The listing builds one solid part. Answer for the finished solid, in the listing's coordinates (mm). Coordinates: 2 decimals unless noted, no trailing zeros. Order: outer loops, then holes, each group sorted by start corner. A loop starts at its lowest first (then second) coordinate and runs counter-clockwise, first axis right, second up. Notation, with made-up numbers: (-21, 89.5) -> (-4, 89.5) arc R11 cw to (-4, 96.5) -> close; hole circle Ø8 at (57.5, 43.5). An arc over 180 degrees is marked (long way). One line per question, with ' | ' between items.
from build123d import *

# Parameters (mm, degrees)
F0_W     = 50.8
F0_H     = 19.05
F1_DEPTH = 1123.95
F2_W     = 122.435573
F2_H     = 50.8
F2_W_2   = 108.831619
F2_W_3   = 93.867282
F2_W_4   = 145.562325
F2_W_5   = 343.160421
F2_W_6   = 239.549167
F3_DEPTH = 25.4
F4_R     = 4.7625
F5_DEPTH = 25.4


with BuildPart() as f1:
    # F0 (on Top) → F1 (new body)
    with BuildSketch(Plane.XY):
        Rectangle(F0_W, F0_H)
    extrude(amount=F1_DEPTH)

    # F2 (on Front) → F3 (cut)
    with BuildSketch(Plane.XZ):
        with Locations((22.446524, 25.4)):
            Rectangle(F2_W, F2_H)
        with Locations((-4.761385, 342.9)):
            Rectangle(F2_W_2, F2_H)
        with Locations((2.720783, 755.65)):
            Rectangle(F2_W_3, F2_H)
        with Locations((-1.360391, 444.5)):
            Rectangle(F2_W_4, F2_H)
        with Locations((-38.781822, 1098.55)):
            Rectangle(F2_W_5, F2_H)
        with Locations((-25.794175, 254)):
            Rectangle(F2_W_6, F2_H)
    extrude(amount=F3_DEPTH, mode=Mode.SUBTRACT)

    # F4 (on Front) → F5 (cut)
    with BuildSketch(Plane.XZ):
        with Locations((15.875, 254)):
            Circle(F4_R)
        with Locations((15.875, 482.6)):
            Circle(F4_R)
    extrude(amount=F5_DEPTH, mode=Mode.SUBTRACT)


solid = f1.part
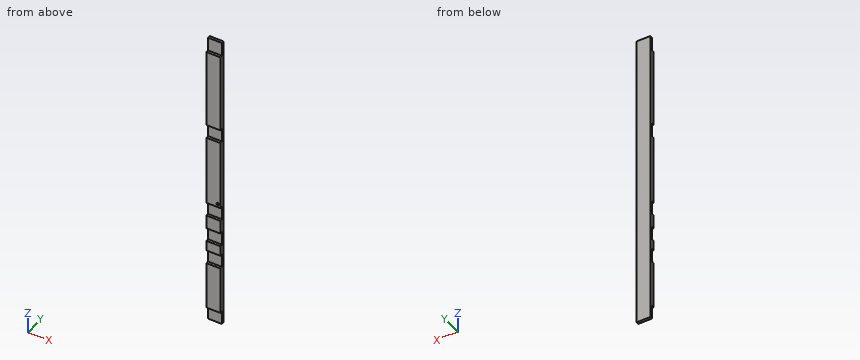
Item 1: Each of these flat-tipped pins is pushed along its axis until it touches: pin 1 Ø4 at (x, y) = (16.5, -4) entering from -Z; pin 2 Ø2 at (x, z) = (-18.5, 430) entering from -Y; pin 3 Ø3 at (x, y) = (12.5, -7) entering from +Z. Where does it stop, or does it pass through?
Computed values:
pin 1: stops at z = 50.8 | pin 2: stops at y = 0 | pin 3: stops at z = 1073.15
Item 2: Section A-A, the plane y = -5.25 is taken. Count the separate pieces of the cut face and the enclosed holes in it, plus the area to 3 significant figures.
Computed values:
separate pieces: 5 | enclosed holes: 1 | area: 41,500 mm^2
Item 3: Section C-C, the plane z = 752.5 is taken. Give the vertices of the cut face in (x, y) (3 decimals).
Computed values:
outline: (-25.4, 0) -> (25.4, 0) -> (25.4, 9.525) -> (-25.4, 9.525) -> close
Item 4: Section B-B, the plane x = -17 is taken. Give the vertices of the cut face in (y, z) (3 decimals), plus the area to 3 significant figures.
Computed values:
outline: (-9.525, 50.8) -> (0, 50.8) -> (0, 0) -> (9.525, 0) -> (9.525, 1123.95) -> (0, 1123.95) -> (0, 1073.15) -> (-9.525, 1073.15) -> (-9.525, 781.05) -> (0, 781.05) -> (0, 730.25) -> (-9.525, 730.25) -> (-9.525, 469.9) -> (0, 469.9) -> (0, 419.1) -> (-9.525, 419.1) -> (-9.525, 368.3) -> (0, 368.3) -> (0, 317.5) -> (-9.525, 317.5) -> (-9.525, 279.4) -> (0, 279.4) -> (0, 228.6) -> (-9.525, 228.6) -> close | area: 18,500 mm^2
Item 5: Find the intervals of material crossed by L1, parallel to Z at x = 22, y = -1.75; L2, parallel to X at y = -3.5, z = 482.6; L3, parallel to Z at x = 12, y = -0.5, in increasing order.
Computed values:
L1: z = 50.8 to 228.6, 279.4 to 317.5, 368.3 to 419.1, 469.9 to 730.25, 781.05 to 1073.15 | L2: x = -25.4 to 11.11, 20.64 to 25.4 | L3: z = 50.8 to 228.6, 279.4 to 317.5, 368.3 to 419.1, 469.9 to 479.83, 485.37 to 730.25, 781.05 to 1073.15
